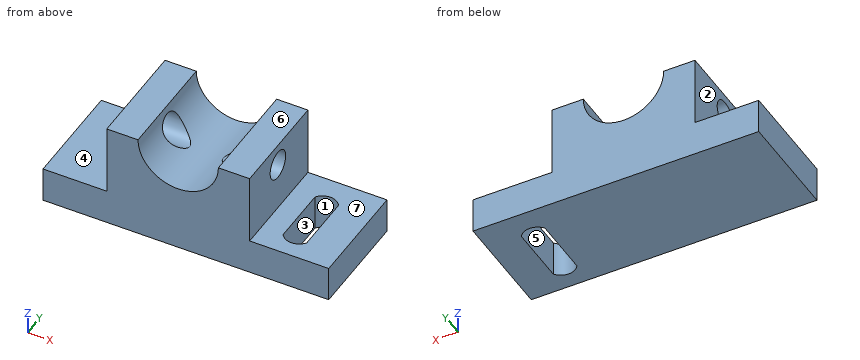
```python
from build123d import *

# Parameters (mm, degrees)
F0_W     = 80
F0_H     = 39.8877346888
F1_DEPTH = 60
F3_DEPTH = 60.001
F5_DEPTH = 20.001
F6_R     = 8
F7_DEPTH = 115.7102386484


# Not quite as in the source:
# - a feature names something its author has since deleted; it is built from what else it names


with BuildPart() as f1:
    # F0 (on Front) → F1 (new body)
    with BuildSketch(Plane.XZ):
        with Locations((0, -35.378112942)):
            Rectangle(F0_W, F0_H)
        Polygon((-75.7092386484, -55.3219802864), (-75.7092386484, -75.3219802864), (84.2907613516, -75.3219802864), (84.2907613516, -55.3219802864), (40, -55.3219802864), (-40, -55.3219802864), align=None)
    extrude(amount=F1_DEPTH)

    # F2 (on face) → F3 (cut, through all)
    with BuildSketch(Plane.XZ.offset(60)):
        with BuildLine():
            Line((-22.5, -15.4342455976), (22.5, -15.4342455976))
            ThreePointArc((22.5, -15.4342455976), (0, 7.0657544024), (-22.5, -15.4342455976))
        make_face()
        with BuildLine():
            ThreePointArc((-22.5, -15.4342455976), (0, -37.9342455976), (22.5, -15.4342455976))
            Line((22.5, -15.4342455976), (-22.5, -15.4342455976))
        make_face()
    extrude(amount=-F3_DEPTH, mode=Mode.SUBTRACT)

    # F4 (on face) → F5 (cut, through all)
    with BuildSketch(Plane.XY.offset(-55.3219802864)):
        with BuildLine():
            Line((65.3745657473, -47.8825420141), (65.3745657473, -15.0121450424))
            ThreePointArc((65.3745657473, -15.0121450424), (58.7502594426, -11.4975174886), (52.1259531379, -15.0121450424))
            Line((52.1259531379, -15.0121450424), (52.1259531379, -47.8825420141))
            ThreePointArc((52.1259531379, -47.8825420141), (58.7502594426, -51.3971695679), (65.3745657473, -47.8825420141))
        make_face()
    extrude(amount=-F5_DEPTH, mode=Mode.SUBTRACT)

    # F6 (on face) → F7 (cut, through all)
    with BuildSketch(Plane.YZ.offset(40)):
        with Locations((-30.8821926572, -27.8876808805)):
            Circle(F6_R)
    extrude(amount=-F7_DEPTH, mode=Mode.SUBTRACT)


solid = f1.part
```
Source: CAD feature listing. Evaluate the final solid. Frame: model axes, mm. Face numbers are marked on the shaded views. A direction names the side the tool comes from. Round coordinates to 2 decimals unless told otherwise and drop trailing zeros. Loops run counter-clockwise (first coordinate to the right, second up) from the corner with the lowest first, then second, coordinate; pieces in that order, holes last. Notation, with made-up numbers: M 30.25,-4 L 59.25,-4 A21 ccw 59.25,33 Z; hole C 25.5,81.5 d2. An arc over 180 degrees is marked long. Put each result on its own line as item: value.
(1) First-contact query: pin 1 (12 mm diameter, centred on y = -32.5, z = -42.5, fed in from -X); pin 2 (12 mm diameter, centred on x = -2, y = -46.5, fed in from +Z); pin 3 (6 mm diameter, centred on x = -53, y = -51, fed in from +Z). Flat tips, straight axial feed; report the tip coordinate or a pass-through.
Solutions:
pin 1: x = -40
pin 2: z = -36.46
pin 3: z = -55.32
(2) Access query for the marked faces 5, 6 and 7. Directions: +Z, -Z, +X, -X, +Y, -Y. A direction counts if a zero-diameter tool reaches every point of the face in a straight line with its end or side. Return the directions, or none.
Solutions:
face 5: +Z, -Z
face 6: +Z, +X, -X, +Y, -Y
face 7: +Z, +X, +Y, -Y
(3) Pull-direction query (X, two-part tool) for the marked faces 1, 2, 3 and 4; classes: released by +X, released by -X, zero draft, split by the parting line, or undercut.
Solutions:
face 1: undercut
face 2: released by -X
face 3: undercut
face 4: zero draft
(4) Section A-A, the plane y = -41. Return loops of the section in (x, z), and give its area (3 significant figures).
Solutions:
outline: M -75.71,-75.32 L 52.13,-75.32 L 52.13,-55.32 L 40,-55.32 L 40,-15.43 L 22.5,-15.43 A22.5 cw -22.5,-15.43 L -40,-15.43 L -40,-55.32 L -75.71,-55.32 Z; M 65.37,-75.32 L 84.29,-75.32 L 84.29,-55.32 L 65.37,-55.32 Z
area: 5,330 mm²
(5) Section C-C, the plane x = 59. Return loops of the section in (y, z).
Solutions:
outline: M -60,-75.32 L -51.39,-75.32 L -51.39,-55.32 L -60,-55.32 Z; M -11.5,-75.32 L 0,-75.32 L 0,-55.32 L -11.5,-55.32 Z
(6) Ray query, line 1 (X direction, y = -20, z = -71); line 2 (X direction, y = -7, z = -43); line 3 (Z direction, x = -59, y = -45). Return the intervals inside material, ascending. Write a range as [from, to].
Solutions:
line 1: [-75.71, 52.13], [65.37, 84.29]
line 2: [-40, 40]
line 3: [-75.32, -55.32]
(7) Section B-B, the plane z = -70.5. Return loops of the section in (x, y), and give its area (3 significant figures).
Solutions:
outline: M -75.71,-60 L 84.29,-60 L 84.29,0 L -75.71,0 Z; hole M 52.13,-47.88 A8 ccw 65.37,-47.88 L 65.37,-15.01 A8 ccw 52.13,-15.01 Z
area: 9,100 mm²
(8) Section D-D, the plane y = -54. Return loops of the section in (x, z).
Solutions:
outline: M -75.71,-75.32 L 84.29,-75.32 L 84.29,-55.32 L 40,-55.32 L 40,-15.43 L 22.5,-15.43 A22.5 cw -22.5,-15.43 L -40,-15.43 L -40,-55.32 L -75.71,-55.32 Z
